Geometry: final body of the model. Coordinates: model frame, mm. A direction names the side the tool comes from. Round coordinates to 2 decimals unless told otherwise and drop trailing zeros. Write each loop counter-clockwise with the first axis right and the second up, starting at its lowest first coordinate (ties: lowest second). Pieces come first, ordered by that corner, then holes. Notation, with made-up numbers: M 85.25,29.5 L 141.25,29.5 A16 cw 141.25,57.5 Z; hole C 13,-32 d11. An arc over 180 degrees is marked long. Use one line per item in the form item = value. Start each with the question number.
Item 1: Section query C-C (y = 4). Return loops of the section in (x, z).
Item 2: Section query B-B (x = 3.5). Return loops of the section in (y, z), and give its area (3 significant figures).
Item 3: Ray query, probe 1 along Y at (x, z) = (0, 12.75); probe 2 along Y at (x, z) = (3, 15.5); probe 3 along X at (y, z) = (-2, 21.25). Return the intervals inside material, ascending.
Item 4: Pull-direction query (Y, two-part tool) for faces 1 (the flat face through (8, 0, 12)), 2 (the cylindrical face through (-1.08, -4.88, 12.32)), 3 (the flat face through (6, 0, 0)), 4 (the flat face through (4, -7, 12)); classes: pulls with the +Y half, pulls with the -Y half, needs draft (parallel to the pull), parting line crosses it, or undercut.
Item 5: Section query D-D (x = 21.5). Return loops of the section in (y, z), and give its area (3 significant figures).
Item 6: Pin query (flat end, axial travel): pin 1 Ø5 at (y, z) = (0.5, 20.5) entering from +X; pin 2 Ø5 at (y, z) = (-1.5, 12.5) entering from +X; pin 3 Ø1 at (x, z) = (18.5, 18) entering from +Y; pin 4 Ø6 at (x, y) = (26, 3.5) entering from +Z. Return the tip coordinate at first contact, or that it passes through.
Item 7: Section query A-A (z = 2.25). Return loops of the section in (x, y).
Item 8: Reachability of faces 5 (the cylindrical face through (21.56, 1.5, 7.73)), 6 (the flat face through (6, 0, 25)) from +Z, -Z, +X, -X, +Y, -Y: full face, straight path, thin tool, end or side. Return the list, or none.
from build123d import *

# Parameters (mm, degrees)
SZKIC1_R                    = 5
DODANIE_WYCI_GNI_CIE1_DEPTH = 25
SZKIC2_R                    = 7
SZKIC2_R_2                  = 5
DODANIE_WYCI_GNI_CIE2_DEPTH = 27.5


with BuildPart() as part:
    # Szkic1 → Dodanie-wyciągnięcie1 (new body)
    with BuildSketch(Plane.XY):
        with BuildLine():
            Line((0, 7), (8, 7))
            Line((8, 7), (8, -7))
            Line((8, -7), (0, -7))
            ThreePointArc((0, -7), (-7, 0), (0, 7))
        make_face()
        Circle(SZKIC1_R, mode=Mode.SUBTRACT)
    extrude(amount=DODANIE_WYCI_GNI_CIE1_DEPTH)

    # Szkic2 → Dodanie-wyciągnięcie2 (add)
    with BuildSketch(Plane(origin=(8, 0, 0), x_dir=(0, 0, -1), z_dir=(1, 0, 0))):
        with Locations(Location((-12.5, 0, 0), (0, 0, 270))):
            Circle(SZKIC2_R)
        with Locations((-12.5, 0)):
            Circle(SZKIC2_R_2, mode=Mode.SUBTRACT)
    extrude(amount=DODANIE_WYCI_GNI_CIE2_DEPTH)


solid = part.part
Working result:
q1.outline = M -5.74,0 L -3,0 L -3,25 L -5.74,25 Z; M 3,0 L 8,0 L 8,6.76 L 35.5,6.76 L 35.5,9.5 L 8,9.5 L 8,15.5 L 35.5,15.5 L 35.5,18.24 L 8,18.24 L 8,25 L 3,25 Z
q2.outline = M -7,0 L -3.57,0 L -3.57,25 L -7,25 Z; M 3.57,0 L 7,0 L 7,25 L 3.57,25 Z
q2.area = 171 mm²
q3.probe_1 = -7 to -5, 5 to 7
q3.probe_2 = -7 to -4, 4 to 7
q3.probe_3 = -6.71 to -4.58, 4.58 to 8
q4.face_1 = undercut
q4.face_2 = undercut
q4.face_3 = needs draft
q4.face_4 = pulls with the -Y half
q5.outline = C 0,12.5 d14; hole C 0,12.5 d10
q5.area = 75.4 mm²
q6.pin_1 = 35.5
q6.pin_2 = 8
q6.pin_3 = 4.9
q6.pin_4 = 19.48
q7.outline = M 0,-7 L 8,-7 L 8,7 L 0,7 A7 ccw Z; hole C 0,0 d10
q8.face_5 = +X
q8.face_6 = +Z, +X, -X, +Y, -Y
